from build123d import *

# Parameters (mm, degrees)
PAD_DEPTH         = 100
SKETCH001_R       = 1.6
SKETCH001_R_2     = 3
POCKET_DEPTH      = 2.001
POCKET_DEPTH_BACK = 2.001
SKETCH004_R       = 11
SKETCH003_R       = 9
SKETCH005_R       = 11
FILLET_R          = 4
FILLET001_R       = 3


with BuildPart() as part:
    # Sketch → Pad (new body)
    with BuildSketch(Plane.YZ):
        Polygon((0, 2), (-20, 2), (-20, 0), (-20, -2), (0, -2), (20, -2), (20, 0), (20, 2), align=None)
    extrude(amount=PAD_DEPTH)

    # Sketch001 → Pocket (cut, two sides)
    with BuildSketch(Plane.XY) as pocket_sk:
        with Locations((14.5, 15.5)):
            Circle(SKETCH001_R)
        with Locations((45.5, 15.5)):
            Circle(SKETCH001_R)
        with Locations((45.5, -15.5)):
            Circle(SKETCH001_R)
        with Locations((14.5, -15.5)):
            Circle(SKETCH001_R)
        with Locations((30, 0)):
            Circle(SKETCH001_R_2)
        with Locations((4, 16)):
            Circle(SKETCH001_R)
        with Locations((4, -16)):
            Circle(SKETCH001_R)
        with Locations((96, 16)):
            Circle(SKETCH001_R)
        with Locations((96, -16)):
            Circle(SKETCH001_R)
    extrude(amount=-POCKET_DEPTH, mode=Mode.SUBTRACT)
    extrude(pocket_sk.sketch, amount=POCKET_DEPTH_BACK, mode=Mode.SUBTRACT)

    # Sketch004 (on DatumPlane) → SubtractiveLoft section 0
    with BuildSketch(Plane.XY.offset(2)):
        with Locations((63, 0)):
            Circle(SKETCH004_R)
    # Sketch003 → SubtractiveLoft section 1
    with BuildSketch(Plane.XY):
        with Locations((63, 0)):
            Circle(SKETCH003_R)
    # Sketch005 (on DatumPlane) → SubtractiveLoft section 2
    with BuildSketch(Plane.XY.offset(-2)):
        with Locations((63, 0)):
            Circle(SKETCH005_R)
    loft(ruled=True, mode=Mode.SUBTRACT)

    # Sketch007 (on DatumPlane) → SubtractiveLoft001 section 0
    with BuildSketch(Plane.XY.offset(2)):
        Polygon((63, 0), (63, 11), (113, 11), (113, -11), (63, -11), align=None)
    # Sketch006 → SubtractiveLoft001 section 1
    with BuildSketch(Plane.XY):
        Polygon((63, 0), (63, 9), (113, 9), (113, -9), (63, -9), align=None)
    # Sketch008 (on DatumPlane) → SubtractiveLoft001 section 2
    with BuildSketch(Plane.XY.offset(-2)):
        Polygon((63, 11), (63, 0), (63, -11), (113, -11), (113, 11), align=None)
    loft(ruled=True, mode=Mode.SUBTRACT)

    # Sketch009 (on DatumPlane) → Groove (revolve, cut)
    with BuildSketch(Plane(origin=(30, 0, 0), x_dir=(1, 0, 0), z_dir=(0, 1, 0))):
        Polygon((4.2, -2), (4.2, 1), (6.638095, -1.4), (6.638095, 1), (9.07619, -1.4), (9.07619, 1), (11.514286, -1.4), (11.514286, 1), (13.952381, -1.4), (13.952381, 1), (17, -2), align=None)
    revolve(axis=Axis((30, 0, 0), (0, 0, -1)), mode=Mode.SUBTRACT)

    # Fillet
    fillet_edges = [part.edges().sort_by_distance(p)[0] for p in [
        (0, -20, 1),
        (0, 20, 1),
        (100, 20, 1),
        (100, -20, 1),
    ]]
    fillet(fillet_edges, radius=FILLET_R)

    # Fillet001
    fillet001_edges = [part.edges().sort_by_distance(p)[0] for p in [
        (100, -10, 1),
        (100, 10, 1),
        (100, 10, -1),
        (100, -10, -1),
    ]]
    fillet(fillet001_edges, radius=FILLET001_R)


solid = part.part
The model under review builds one solid part; all positions refer to its coordinate system, in mm. A direction names the side the tool comes from. Round coordinates to 2 decimals unless told otherwise and drop trailing zeros. Loops run counter-clockwise (first coordinate to the right, second up) from the corner with the lowest first, then second, coordinate; pieces in that order, holes last. Notation, with made-up numbers: (61, 13.25) -> (75, 13.25) arc R11 ccw to (75, 33.25) -> close; hole circle Ø10 at (79.5, 52). An arc over 180 degrees is marked (long way). Write item = value, one per line. Start each with the question number.
Item 1: Mouldability with a two-part tool opening along Y and no side actions: class faces 4 (the flat face through (100, -15, 0)), 5 (the cylindrical face through (29.09, 4.1, 0.48)), 6 (the flat face through (49, 20, 0)) as released by +Y, released by -Y, zero draft, split by the parting line, or undercut.
Item 2: Take a section at C-C on x = 45.5. Count the separate pieces of the cut face and the enclosed holes in it, plus the area to 3 significant figures.
Item 3: For faces 1 (the flat face through (80, 10, 1)), 2 (the flat face through (0, 0, 0)), 3 (the flat face through (80, 10, -1)), list the 3-axis set-ups (+Z, -Z, +X, -X, +Y, -Y) from which the entire face can be reached by the end or side of a thin tool; tool diameter is ignored.
Item 4: To check wall thickness, follow L1, parallel to Y at x = 4, z = 0.9; L2, parallel to Y at x = 14.5, z = -0.55; L3, parallel to Y at x = 96, z = 1. State the ranges of each line that lie inside material, in increasing order.
Item 5: Take a section at A-A on x = 80. Give the boundary of the cut face in (y, z), plus the area to 3 significant figures.
Result:
q1.face_4 = zero draft
q1.face_5 = undercut
q1.face_6 = released by +Y
q2.separate_pieces = 3
q2.enclosed_holes = 0
q2.area = 121 mm²
q3.face_1 = +Z, +X
q3.face_2 = +Z, -Z, -X, +Y, -Y
q3.face_3 = -Z, +X
q4.L1 = -20 to -17.6, -14.4 to 14.4, 17.6 to 20
q4.L2 = -20 to -17.1, -13.9 to 13.9, 17.1 to 20
q4.L3 = -20 to -17.6, -14.4 to -10, 10 to 14.4, 17.6 to 20
q5.outline = (-20, -2) -> (-11, -2) -> (-9, 0) -> (-11, 2) -> (-20, 2) -> close; (9, 0) -> (11, -2) -> (20, -2) -> (20, 2) -> (11, 2) -> close
q5.area = 80.0 mm²
